Could you check a few things on this model? Use its own coordinates, in mm. Give positions to 0.01 mm unless a question says otherwise; leave off trailing zeros. Write each loop counter-clockwise with the first axis right and the second up, starting at its lowest first coordinate (ties: lowest second). Pieces come first, ordered by that corner, then holes. Notation, with made-up numbers: (84.5, 18) - (104.5, 18) arc R6 ccw to (104.5, 29) - close; hole circle Ø3 at (15.25, 68.25). An arc over 180 degrees is marked (long way). Write item = value, one per line.
from build123d import *

# Parameters (mm, degrees)
SKETCH1_R           = 5.08
BOSS_EXTRUDE1_DEPTH = 6.985
CUT_EXTRUDE1_DEPTH  = 4.445
SKETCH3_R           = 3.175
CUT_EXTRUDE2_DEPTH  = 2.54


with BuildPart() as part:
    # Sketch1 → Boss-Extrude1 (new body)
    with BuildSketch(Plane(origin=(0, 0, 0), x_dir=(1, 0, 0), z_dir=(0, 1, 0))):
        Circle(SKETCH1_R)
    extrude(amount=BOSS_EXTRUDE1_DEPTH)

    # Sketch2 → Cut-Extrude1 (cut)
    with BuildSketch(Plane(origin=(0, 0, 0), x_dir=(1, 0, 0), z_dir=(0, 1, 0))):
        with BuildLine():
            Line((-2.7178, 1.941605307), (-2.7178, -1.941605307))
            ThreePointArc((-2.7178, -1.941605307), (1.019446965, -3.180722543), (3.3401, 0))
            ThreePointArc((3.3401, 0), (1.019446965, 3.180722543), (-2.7178, 1.941605307))
        make_face()
    extrude(amount=CUT_EXTRUDE1_DEPTH, mode=Mode.SUBTRACT)

    # Sketch3 → Cut-Extrude2 (cut)
    with BuildSketch(Plane(origin=(0, 6.985, 0), x_dir=(1, 0, 0), z_dir=(0, 1, 0))):
        Circle(SKETCH3_R)
    extrude(amount=-CUT_EXTRUDE2_DEPTH, mode=Mode.SUBTRACT)


solid = part.part
1. If we section it at C-C, the plane y = 4.75: Please give me the cut outline in (x, z) (3 decimals), and give its area (3 significant figures).
Filled sheet:
outline = circle Ø10.16 at (0, 0); hole circle Ø6.35 at (0, 0)
area = 49.4 mm2
2. I need wall thicknesses on line 1 (X direction, y = 6.1, z = 0) (3 decimals); line 2 (X direction, y = 5.5, z = -1.75). Which ranges of each line are inside material? Lowest first, please.
Filled sheet:
line_1 = -5.08 to -3.175, 3.175 to 5.08
line_2 = -4.77 to -2.65, 2.65 to 4.77
3. If we section it at B-B, the plane z = -2.75: Please give me the cut outline in (x, y) (3 decimals).
Filled sheet:
outline = (-4.271, 0) - (-1.896, 0) - (-1.896, 4.445) - (-1.587, 4.445) - (-1.587, 6.985) - (-4.271, 6.985) - close; (1.587, 4.445) - (1.896, 4.445) - (1.896, 0) - (4.271, 0) - (4.271, 6.985) - (1.587, 6.985) - close
4. If we section it at A-A, the plane x = 0: Please give me the cut outline in (y, z) (3 decimals).
Filled sheet:
outline = (0, -5.08) - (6.985, -5.08) - (6.985, -3.175) - (4.445, -3.175) - (4.445, -3.34) - (0, -3.34) - close; (0, 3.34) - (4.445, 3.34) - (4.445, 3.175) - (6.985, 3.175) - (6.985, 5.08) - (0, 5.08) - close
5. Thinking about a two-plate mould opening in Z: for faces 1 (the face through (3.3, 6.985, 1.1)), 2 (the face through (-2.718, 2, 0)), 3 (the face through (-0.661, 3.444, -5.037)), 4 (the face through (-0.69, 5.73, 3.1)), which applies, pulls with the +Z half, pulls with the -Z half, needs draft (parallel to the pull), parting line crosses it, or undercut?
Filled sheet:
face_1 = needs draft
face_2 = undercut
face_3 = parting line crosses it
face_4 = undercut
6. For pin 1 (1 mm diameter, centred on y = 1.5, z = 3.5, fed in from -X); pin 2 (4 mm diameter, centred on x = 0, z = 0, fed in from +Y); pin 3 (2 mm diameter, centred on y = 4, z = 2, fed in from -X), each with a flat end and sliding along its axis, tell me the tip position at first contact or that it passes through.
Filled sheet:
pin_1 = -4.1
pin_2 = through
pin_3 = -4.98
7. If we section it at D-D, the plane y = 1.5: Please give me the cut outline in (x, z).
Filled sheet:
outline = circle Ø10.16 at (0, 0); hole (-2.72, -1.94) arc R3.34 ccw (long way) to (-2.72, 1.94) - close
